Geometry check sheet. Reference: the model listing, model coordinates, mm. A direction names the side the tool comes from. Round coordinates to 2 decimals unless told otherwise and drop trailing zeros. Order: outer loops, then holes, each group sorted by start corner. A loop starts at its lowest first (then second) coordinate and runs counter-clockwise, first axis right, second up. Notation, with made-up numbers: (18, 85) - (49, 85) arc R12 ccw to (49, 98) - close; hole circle Ø3 at (84, -10). An arc over 180 degrees is marked (long way). Write each question's results on one line, items separated by ' | '.
```python
from build123d import *

# Parameters (mm, degrees)
F0_R     = 1.5875
F0_R_2   = 3.175
F1_DEPTH = 3.048
F3_DEPTH = 25.4


with BuildPart() as f1:
    # F0 (on Front) → F1 (new body)
    with BuildSketch(Plane.XZ):
        with BuildLine():
            ThreePointArc((0, -15.875), (11.2253201513, -11.2253201513), (15.875, 0))
            ThreePointArc((15.875, 0), (15.8430821306, 1.0061677811), (15.7474568688, 2.0082896118))
            ThreePointArc((15.7474568688, 2.0082896118), (10.4912827484, 11.9142188705), (0, 15.875))
            Line((0, 15.875), (0, 3.175))
            ThreePointArc((0, 3.175), (2.2450640303, 2.2450640303), (3.175, 0))
            ThreePointArc((3.175, 0), (2.2450640303, -2.2450640303), (0, -3.175))
            Line((0, -3.175), (0, -15.875))
        make_face()
        with BuildLine():
            ThreePointArc((15.7474568688, 2.0082896118), (15.8430821306, 1.0061677811), (15.875, 0))
            ThreePointArc((15.875, 0), (11.2253201513, -11.2253201513), (0, -15.875))
            Line((0, -15.875), (0, -53.975))
            ThreePointArc((0, -53.975), (6.7351920908, -56.7648079092), (9.525, -63.5))
            ThreePointArc((9.525, -63.5), (6.9712901065, -69.9905114784), (0.6794904459, -73.0007324841))
            Line((0.6794904459, -73.0007324841), (44.45, -71.4375))
            ThreePointArc((44.45, -71.4375), (36.5125, -63.5), (44.45, -55.5625))
            Line((44.45, -55.5625), (18.8464820385, -55.5625))
            add(Edge.make_bspline(
                [(18.8464820385, -55.5625), (16.9357606523, -55.0097091598), (9.4372158473, -52.8403050213), (13.1997682789, -22.5625848825), (16.0035761028, 0)],
                knots=[0, 0, 0, 0, 0.2548122917, 1, 1, 1, 1], degree=3))
            Line((16.0035761028, 0), (15.7474568688, 2.0082896118))
        make_face()
        with BuildLine():
            ThreePointArc((0, 15.875), (10.4912827484, 11.9142188705), (15.7474568688, 2.0082896118))
            Line((15.7474568688, 2.0082896118), (9.525, 50.8))
            ThreePointArc((9.525, 50.8), (6.7351920908, 44.0648079092), (0, 41.275))
            Line((0, 41.275), (0, 15.875))
        make_face()
        with BuildLine():
            Line((0, -53.975), (0, -15.875))
            ThreePointArc((0, -15.875), (-10.634629101, -11.7864451335), (-15.7914295954, -1.6267686783))
            Line((-15.7914295954, -1.6267686783), (-9.4772560787, -64.4524926348))
            ThreePointArc((-9.4772560787, -64.4524926348), (-7.0639265761, -57.1104330094), (0, -53.975))
        make_face()
        with BuildLine():
            ThreePointArc((-15.7914295954, -1.6267686783), (-10.634629101, -11.7864451335), (0, -15.875))
            Line((0, -15.875), (0, -3.175))
            ThreePointArc((0, -3.175), (-3.175, 0), (0, 3.175))
            Line((0, 3.175), (0, 15.875))
            ThreePointArc((0, 15.875), (-10.4912827447, 11.9142188737), (-15.7474568676, 2.0082896216))
            ThreePointArc((-15.7474568676, 2.0082896216), (-15.8738386045, 0.192023326), (-15.7914295954, -1.6267686783))
        make_face()
        with BuildLine():
            ThreePointArc((-15.7474568676, 2.0082896216), (-10.4912827447, 11.9142188737), (0, 15.875))
            Line((0, 15.875), (0, 41.275))
            ThreePointArc((0, 41.275), (-6.7351920908, 44.0648079092), (-9.525, 50.8))
            Line((-9.525, 50.8), (-15.7474568676, 2.0082896216))
        make_face()
        with Locations((-1.9409962697, 36.5252)):
            Circle(F0_R, mode=Mode.SUBTRACT)
        with BuildLine():
            ThreePointArc((0, 41.275), (6.7351920908, 44.0648079092), (9.525, 50.8))
            ThreePointArc((9.525, 50.8), (0, 60.325), (-9.525, 50.8))
            ThreePointArc((-9.525, 50.8), (-6.7351920908, 44.0648079092), (0, 41.275))
        make_face()
        with BuildLine():
            ThreePointArc((3.175, 50.8), (2.2450640303, 48.5549359697), (0, 47.625))
            ThreePointArc((0, 47.625), (-2.2450640303, 53.0450640303), (3.175, 50.8))
        make_face(mode=Mode.SUBTRACT)
        with BuildLine():
            ThreePointArc((9.525, -63.5), (6.7351920908, -56.7648079092), (0, -53.975))
            ThreePointArc((0, -53.975), (-7.0639265761, -57.1104330094), (-9.4772560787, -64.4524926348))
            ThreePointArc((-9.4772560787, -64.4524926348), (-6.3895669906, -70.5639265761), (0, -73.025))
            Line((0, -73.025), (0.6794904459, -73.0007324841))
            ThreePointArc((0.6794904459, -73.0007324841), (6.9712901065, -69.9905114784), (9.525, -63.5))
        make_face()
        with BuildLine():
            ThreePointArc((3.175, -63.5), (-2.2450640303, -65.7450640303), (0, -60.325))
            ThreePointArc((0, -60.325), (2.2450640303, -61.2549359697), (3.175, -63.5))
        make_face(mode=Mode.SUBTRACT)
        with BuildLine():
            ThreePointArc((52.3875, -63.5), (50.0626600757, -57.8873399243), (44.45, -55.5625))
            ThreePointArc((44.45, -55.5625), (36.5125, -63.5), (44.45, -71.4375))
            ThreePointArc((44.45, -71.4375), (50.0626600757, -69.1126600757), (52.3875, -63.5))
        make_face()
        with Locations((44.45, -63.5)):
            Circle(F0_R_2, mode=Mode.SUBTRACT)
        with BuildLine():
            Line((0.6794904459, -73.0007324841), (0, -73.025))
            ThreePointArc((0, -73.025), (0.3399618281, -73.0189311877), (0.6794904459, -73.0007324841))
        make_face()
    extrude(amount=F1_DEPTH)

    # F2 (on Front) → F3 (join)
    with BuildSketch(Plane.XZ):
        Polygon((42.2361642122, 49.5914518833), (-25.550276041, 49.5914518833), (-25.550276041, 0), (42.2361642122, 0), (42.2361642122, 47.7479062974), align=None)
    extrude(amount=F3_DEPTH)


solid = f1.part
```
(1) Material ranges on line 1 (X direction, y = -0.85, z = 50.8) (3 decimals); line 2 (X direction, y = -21, z = 13); line 3 (Y direction, x = 12.5, z = -15), recorded low to high.
Answers follow:
line 1: -9.525 to -3.175, 3.175 to 9.525 | line 2: -25.55 to 42.24 | line 3: -3.05 to 0
(2) Section check A-A (x = 30). Record the cut outline in (y, z).
Answers follow:
outline: (-25.4, 0) - (0, 0) - (0, 49.59) - (-25.4, 49.59) - close; (-3.05, -71.95) - (0, -71.95) - (0, -55.56) - (-3.05, -55.56) - close
(3) Depth check by flat-ended pin: pin 1 Ø2 at (y, z) = (-16, 39) entering from +X; pin 2 Ø12.5 at (x, y) = (5, -18.5) entering from -Z; pin 3 Ø8.5 at (x, z) = (1.5, 56) entering from -Y. Enter the tip coordinate at first touch or a pass-through.
Answers follow:
pin 1: x = 42.24 | pin 2: z = 0 | pin 3: y = -3.05
(4) Draft check along Z on faces 1 (the face through (42.236, -13, 24)), 2 (the face through (0.209, -1.503, 60.323)), 3 (the face through (32, -2, -55.562)). Enter one of: released by +Z, released by -Z, zero draft, split by the parting line, or undercut.
Answers follow:
face 1: zero draft | face 2: released by +Z | face 3: undercut
(5) Section check D-D (y = -5.25). Record the cut outline in (x, z), then the cut area to 3 significant figures.
Answers follow:
outline: (-25.55, 0) - (42.24, 0) - (42.24, 49.59) - (-25.55, 49.59) - close | area: 3,360 mm²
(6) Section check B-B (x = 6). Record the cut outline in (y, z).
Answers follow:
outline: (-25.4, 0) - (-3.05, 0) - (-3.05, -72.81) - (0, -72.81) - (0, 58.2) - (-3.05, 58.2) - (-3.05, 49.59) - (-25.4, 49.59) - close
(7) Section check C-C (z = 21). Record the cut outline in (x, y), then the cut area to 3 significant figures.
Answers follow:
outline: (-25.55, -25.4) - (42.24, -25.4) - (42.24, 0) - (-25.55, 0) - close | area: 1,720 mm²
(8) Access from +Z, -Z, +X, -X, +Y, -Y to the whole of each face (thin tool, end or side, straight path). Record for faces 4 (the face through (0, -3.048, 55)), 5 (the face through (-12.68, -1.5, -32.6)), 6 (the face through (10, -3.048, -44)).
Answers follow:
face 4: +Z, +X, -X, -Y | face 5: -Z, -X, +Y, -Y | face 6: -Z, +X, -X, -Y
